```python
from build123d import *

# Parameters (mm, degrees)
SKETCH1_W                    = 76.2
SKETCH1_H                    = 50.8
BOSS_EXTRUDE1_DEPTH          = 114.3
CUT_EXTRUDE2_DEPTH           = 49.022
SKETCH6_R                    = 2.286
CUT_EXTRUDE3_DEPTH           = 5.08
CUT_EXTRUDE3_DRAFT           = -3
CUT_EXTRUDE3_PROFILE_2_DEPTH = 5.08
CUT_EXTRUDE3_PROFILE_2_DRAFT = -3
CUT_EXTRUDE3_PROFILE_3_DEPTH = 5.08
CUT_EXTRUDE3_PROFILE_3_DRAFT = -3
CUT_EXTRUDE3_PROFILE_4_DEPTH = 5.08
CUT_EXTRUDE3_PROFILE_4_DRAFT = -3
SKETCH10_W                   = 15.24
SKETCH10_H                   = 15.24
SKETCH10_W_2                 = 17.018
CUT_EXTRUDE4_DEPTH           = 5.08


with BuildPart() as part:
    # Sketch1 → Boss-Extrude1 (new body)
    with BuildSketch(Plane.XY):
        with Locations((38.1, 10.497687861)):
            Rectangle(SKETCH1_W, SKETCH1_H)
    extrude(amount=BOSS_EXTRUDE1_DEPTH)

    # Sketch3 → Cut-Extrude2 (cut)
    with BuildSketch(Plane.XZ.offset(14.902312139)):
        Polygon((65.532, 112.522), (10.668, 112.522), (10.668, 103.632), (1.778, 103.632), (1.778, 10.668), (10.668, 10.668), (10.668, 1.778), (65.532, 1.778), (65.532, 10.668), (74.422, 10.668), (74.422, 103.632), (65.532, 103.632), align=None)
    extrude(amount=-CUT_EXTRUDE2_DEPTH, mode=Mode.SUBTRACT)


with BuildPart() as cut_extrude3_tool:
    # Sketch6 → Cut-Extrude3 (with draft: the straight prism first)
    with BuildSketch(Plane(origin=(0, -14.902312139, 0), x_dir=(-1, 0, 0), z_dir=(0, -1, 0))):
        with Locations((-69.85, -6.35)):
            Circle(SKETCH6_R)
    extrude(amount=-CUT_EXTRUDE3_DEPTH)
    # Cut-Extrude3: the draft: its side faces are tilted about the plane it starts from
    cut_extrude3_sides = [cut_extrude3_tool.faces().sort_by_distance(p)[0] for p in [
        (72.136, -12.362312139, 6.35),
    ]]
    draft(cut_extrude3_sides, Plane(origin=(0, -14.902312139, 0), x_dir=(-1, 0, 0), z_dir=(0, -1, 0)), CUT_EXTRUDE3_DRAFT)


with BuildPart() as part_1:
    add(part.part)

    # Cut-Extrude3: cut by cut_extrude3_tool
    add(cut_extrude3_tool.part, mode=Mode.SUBTRACT)


with BuildPart() as cut_extrude3_profile_2_tool:
    # Sketch6 → Cut-Extrude3 profile 2 (with draft: the straight prism first)
    with BuildSketch(Plane(origin=(0, -14.902312139, 0), x_dir=(-1, 0, 0), z_dir=(0, -1, 0))):
        with Locations((-6.35, -6.35)):
            Circle(SKETCH6_R)
    extrude(amount=-CUT_EXTRUDE3_PROFILE_2_DEPTH)
    # Cut-Extrude3 profile 2: the draft: its side faces are tilted about the plane it starts from
    cut_extrude3_profile_2_sides = [cut_extrude3_profile_2_tool.faces().sort_by_distance(p)[0] for p in [
        (8.636, -12.362312139, 6.35),
    ]]
    draft(cut_extrude3_profile_2_sides, Plane(origin=(0, -14.902312139, 0), x_dir=(-1, 0, 0), z_dir=(0, -1, 0)), CUT_EXTRUDE3_PROFILE_2_DRAFT)


with BuildPart() as part_2:
    add(part_1.part)

    # Cut-Extrude3 profile 2: cut by cut_extrude3_profile_2_tool
    add(cut_extrude3_profile_2_tool.part, mode=Mode.SUBTRACT)


with BuildPart() as cut_extrude3_profile_3_tool:
    # Sketch6 → Cut-Extrude3 profile 3 (with draft: the straight prism first)
    with BuildSketch(Plane(origin=(0, -14.902312139, 0), x_dir=(-1, 0, 0), z_dir=(0, -1, 0))):
        with Locations((-6.35, -107.95)):
            Circle(SKETCH6_R)
    extrude(amount=-CUT_EXTRUDE3_PROFILE_3_DEPTH)
    # Cut-Extrude3 profile 3: the draft: its side faces are tilted about the plane it starts from
    cut_extrude3_profile_3_sides = [cut_extrude3_profile_3_tool.faces().sort_by_distance(p)[0] for p in [
        (8.636, -12.362312139, 107.95),
    ]]
    draft(cut_extrude3_profile_3_sides, Plane(origin=(0, -14.902312139, 0), x_dir=(-1, 0, 0), z_dir=(0, -1, 0)), CUT_EXTRUDE3_PROFILE_3_DRAFT)


with BuildPart() as part_3:
    add(part_2.part)

    # Cut-Extrude3 profile 3: cut by cut_extrude3_profile_3_tool
    add(cut_extrude3_profile_3_tool.part, mode=Mode.SUBTRACT)


with BuildPart() as cut_extrude3_profile_4_tool:
    # Sketch6 → Cut-Extrude3 profile 4 (with draft: the straight prism first)
    with BuildSketch(Plane(origin=(0, -14.902312139, 0), x_dir=(-1, 0, 0), z_dir=(0, -1, 0))):
        with Locations((-69.85, -107.95)):
            Circle(SKETCH6_R)
    extrude(amount=-CUT_EXTRUDE3_PROFILE_4_DEPTH)
    # Cut-Extrude3 profile 4: the draft: its side faces are tilted about the plane it starts from
    cut_extrude3_profile_4_sides = [cut_extrude3_profile_4_tool.faces().sort_by_distance(p)[0] for p in [
        (72.136, -12.362312139, 107.95),
    ]]
    draft(cut_extrude3_profile_4_sides, Plane(origin=(0, -14.902312139, 0), x_dir=(-1, 0, 0), z_dir=(0, -1, 0)), CUT_EXTRUDE3_PROFILE_4_DRAFT)


with BuildPart() as part_4:
    add(part_3.part)

    # Cut-Extrude3 profile 4: cut by cut_extrude3_profile_4_tool
    add(cut_extrude3_profile_4_tool.part, mode=Mode.SUBTRACT)

    # Sketch10 → Cut-Extrude4 (cut)
    with BuildSketch(Plane(origin=(0, 0, 0), x_dir=(-1, 0, 0), z_dir=(0, 0, -1))):
        with Locations((-55.88, 25.737687861)):
            Rectangle(SKETCH10_W, SKETCH10_H)
        with Locations((-19.751, 25.737687861)):
            Rectangle(SKETCH10_W_2, SKETCH10_H)
    extrude(amount=-CUT_EXTRUDE4_DEPTH, mode=Mode.SUBTRACT)


solid = part_4.part
```
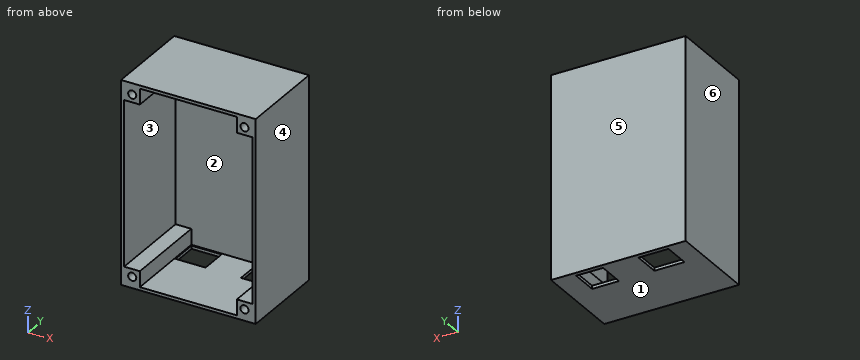
Here's how the part is built. I have some questions about the finished solid (model axes, mm). Face numbers are marked on the shaded views. A direction names the side the tool comes from. Coordinates: 2 decimals unless noted, no trailing zeros. Write each loop counter-clockwise with the first axis right and the second up, starting at its lowest first coordinate (ties: lowest second). Pieces come first, ordered by that corner, then holes. Notation, with made-up numbers: (54.25, -5) -> (100.25, -5) arc R11 cw to (100.25, 11) -> close; hole circle Ø7 at (40.5, -4.75). An arc over 180 degrees is marked (long way). Use a Markdown table: item, result. Add a question column.
(1) If we section it at D-D, the plane y = 15.5: Write out the boundary of the cut face in (x, z), and give its area (3 significant figures).
(2) Please list where these lines run through material, in increasing order: line 1 (Z direction, x = 53.5, y = 9); line 2 (X direction, y = 14.5, z = 77); line 3 (Z direction, x = 6, y = 28).
(3) I'm going to push flat-ended pins straight in: P1, Ø4.5, axis at y = -2.5, z = 106, coming from the -X side; P2, Ø2, axis at x = 69.5, z = 107.5, coming from the -Y side. Where does each tip first touch, or does it pass through?
(4) We'd pull the mould along X, two halves only. Please class the marked faces 3, 4, 5 and 6: +X half, -X half, draft (parallel to the pull), parting line (faces both ways), or undercut.
(5) If we section it at C-C, the plane z = 107.95: Write out the boundary of the cut face in (x, y), and give its area (3 significant figures).
(6) For the marked faces 1 and 2, which set-ups out of +Z, -Z, +X, -X, +Y, -Y let a thin tool reach every point of the face, with its end or its side?
(7) If we section it at B-B, the plane x = 69.85: Write out the boundary of the cut face in (y, z).
(8) If we section it at A-A, the plane y = 24.5: Write out the boundary of the cut face in (x, z), and give its area (3 significant figures).
Outcome:
| question | item | result |
|---|---|---|
| 1 | outline | (0, 0) -> (76.2, 0) -> (76.2, 114.3) -> (0, 114.3) -> close; hole (1.78, 10.67) -> (10.67, 10.67) -> (10.67, 1.78) -> (65.53, 1.78) -> (65.53, 10.67) -> (74.42, 10.67) -> (74.42, 103.63) -> (65.53, 103.63) -> (65.53, 112.52) -> (10.67, 112.52) -> (10.67, 103.63) -> (1.78, 103.63) -> close |
| 1 | area | 981 mm^2 |
| 2 | line 1 | z = 0 to 1.78, 112.52 to 114.3 |
| 2 | line 2 | x = 0 to 1.78, 74.42 to 76.2 |
| 2 | line 3 | z = 0 to 10.67, 103.63 to 114.3 |
| 3 | P1 | stops at x = 0 |
| 3 | P2 | stops at y = -9.82 |
| 4 | face 3 | undercut |
| 4 | face 4 | +X half |
| 4 | face 5 | draft |
| 4 | face 6 | -X half |
| 5 | outline | (0, -14.9) -> (4.06, -14.9) -> (4.33, -9.82) -> (8.37, -9.82) -> (8.64, -14.9) -> (10.67, -14.9) -> (10.67, 34.12) -> (65.53, 34.12) -> (65.53, -14.9) -> (67.56, -14.9) -> (67.83, -9.82) -> (71.87, -9.82) -> (72.14, -14.9) -> (76.2, -14.9) -> (76.2, 35.9) -> (0, 35.9) -> close |
| 5 | area | 1,140 mm^2 |
| 6 | face 1 | -Z, +X, -X, +Y, -Y |
| 6 | face 2 | -Y |
| 7 | outline | (-14.9, 0) -> (35.9, 0) -> (35.9, 114.3) -> (-14.9, 114.3) -> (-14.9, 110.24) -> (-9.82, 109.97) -> (-9.82, 105.93) -> (-14.9, 105.66) -> (-14.9, 103.63) -> (34.12, 103.63) -> (34.12, 10.67) -> (-14.9, 10.67) -> (-14.9, 8.64) -> (-9.82, 8.37) -> (-9.82, 4.33) -> (-14.9, 4.06) -> close |
| 8 | outline | (0, 0) -> (11.24, 0) -> (11.24, 1.78) -> (10.67, 1.78) -> (10.67, 10.67) -> (1.78, 10.67) -> (1.78, 103.63) -> (10.67, 103.63) -> (10.67, 112.52) -> (65.53, 112.52) -> (65.53, 103.63) -> (74.42, 103.63) -> (74.42, 10.67) -> (65.53, 10.67) -> (65.53, 1.78) -> (63.5, 1.78) -> (63.5, 0) -> (76.2, 0) -> (76.2, 114.3) -> (0, 114.3) -> close; (28.26, 0) -> (48.26, 0) -> (48.26, 1.78) -> (28.26, 1.78) -> close |
| 8 | area | 924 mm^2 |
